For this review, take the finished solid that the model builds, in its own axes (mm). A direction names the side the tool comes from. Coordinates: 2 decimals unless noted, no trailing zeros. Order: outer loops, then holes, each group sorted by start corner. A loop starts at its lowest first (then second) coordinate and runs counter-clockwise, first axis right, second up. Notation, with made-up numbers: (84.5, 30) -> (108.5, 30) arc R38 ccw to (108.5, 68) -> close; hole circle Ø3 at (65, 12). An arc over 180 degrees is marked (long way). Return JSON: item names as keys, results as strings. Group by question number.
Item 1: Take a section at B-B (z = -6). Write out the cut boundary in (x, y), then the cut area to 3 significant figures.
Item 2: Take a section at D-D (x = -1). Write out the cut boundary in (y, z), then the cut area to 3 significant figures.
Item 3: Machinability: for faces 5 (the flat face through (0, 10, -5)), 6 (the cylindrical face through (-20.839, -4.213, -5.549)), 7 (the cylindrical face through (-41, 0, 2)), which of the approach directions +Z, -Z, +X, -X, +Y, -Y give a long, thin tool a straight path to every point of the face, cutting with its end or side? Answer none if there is none.
Item 4: Take a section at A-A (x = -31). Write out the cut boundary in (y, z), then the cut area to 4 significant figures.
Item 5: Draft analysis for pull direction Y (two halves, no side actions). For faces 1 (the flat face through (-78, 18.5, -2)), 2 (the flat face through (-4, -13.5, -2)), 3 (the cylindrical face through (-166.33, 16.04, -0.35)), 4 (the flat face through (-29, -10, -2)), state which applies: +Y half, -Y half, draft (parallel to the pull), parting line (faces both ways), or undercut.
Item 6: Take a section at C-C (y = 0). Write out the cut boundary in (x, z).
Item 7: For line 1 along Y through (x, z) = (-12, 4.85); line 2 along X through (y, z) = (16.95, -1.5); line 3 along Y through (x, z) = (-48.5, -8.25), list the stretches that pass through material, from the lowest coordinate up.
Item 8: Insertion check: pin 1 (4.5 mm diameter, centred on x = -6, z = -6, fed in from -Y); pin 2 (2 mm diameter, centred on y = -6, z = 3, fed in from -X); pin 3 (6 mm diameter, centred on x = 4, y = 3.5, fed in from -Z). Each pin has a flat end and moves straight along its axis. Give the tip position at first contact, or say it passes through.
```python
from build123d import *

# Parameters (mm, degrees)
SKETCH_1_W          = 40
SKETCH_1_H          = 20
EXTRUDE_1_DEPTH     = 6
SKETCH_2_R          = 2.5
CUT_EXTRUDE_1_DEPTH = 24.151673806
EXTRUDE_START       = -15
EXTRUDE_2_OUTLINE_R = 11
EXTRUDE_2_DEPTH     = 15
EXTRUDE_START_2     = -8
SKETCH_5_R          = 11
SKETCH_5_R_2        = 10
EXTRUDE_3_DEPTH     = 8
SKETCH_8_W          = 15
SKETCH_8_H          = 5
EXTRUDE_4_DEPTH     = 200
SKETCH_9_W          = 4.403653586
SKETCH_9_H          = 3.736433346
EXTRUDE_5_DEPTH     = 15
SKETCH_13_W         = 64.67728996
SKETCH_13_H         = 18.524474632
CUT_EXTRUDE_2_DEPTH = 184.131783151
SKETCH_15_W         = 55.676477601
SKETCH_15_H         = 15
EXTRUDE_6_DEPTH     = 5
SKETCH_16_R         = 2.5
CUT_EXTRUDE_3_DEPTH = 10


# Read off the part's stored shape, not the designer's step: 凸台-拉伸2
with BuildPart() as part:
    # 草图1 → 凸台-拉伸1 (new body)
    with BuildSketch(Plane.XY):
        Rectangle(SKETCH_1_W, SKETCH_1_H)
    extrude(amount=EXTRUDE_1_DEPTH)

    # 草图2 → 切除-拉伸1 (cut, through all)
    with BuildSketch(Plane.XY.offset(6)):
        with Locations((10, 0)):
            Circle(SKETCH_2_R)
        with Locations((-1, 0)):
            Circle(SKETCH_2_R)
        with Locations((-12, 0)):
            Circle(SKETCH_2_R)
    extrude(amount=-CUT_EXTRUDE_1_DEPTH, mode=Mode.SUBTRACT)

    # 凸台-拉伸2 outline → 凸台-拉伸2 (add)
    with BuildSketch(Plane.XY.offset(6).offset(EXTRUDE_START)):
        with BuildLine():
            Line((20, 10), (20, 13.5))
            Line((20, 13.5), (-26.893967141, 13.5))
            Line((-26.893967141, 13.5), (-26.893967141, 13.384337644))
            ThreePointArc((-26.893967141, 13.384337644), (-45, 0), (-26.893967141, -13.384337644))
            Line((-26.893967141, -13.384337644), (-26.893967141, -13.5))
            Line((-26.893967141, -13.5), (20, -13.5))
            Line((20, -13.5), (20, -10))
            Line((20, -10), (-20, -10))
            Line((-20, -10), (-20, -8.660254038))
            ThreePointArc((-20, -8.660254038), (-17, 0), (-20, 8.660254038))
            Line((-20, 8.660254038), (-20, 10))
            Line((-20, 10), (20, 10))
        make_face()
        with Locations((-31, 0)):
            Circle(EXTRUDE_2_OUTLINE_R, mode=Mode.SUBTRACT)
    extrude(amount=EXTRUDE_2_DEPTH)

    # 草图5 → 凸台-拉伸3 (add)
    with BuildSketch(Plane.XY.offset(6).offset(EXTRUDE_START_2)):
        with Locations((-31, 0)):
            Circle(SKETCH_5_R)
        with Locations((-31, 0)):
            Circle(SKETCH_5_R_2, mode=Mode.SUBTRACT)
    extrude(amount=EXTRUDE_3_DEPTH)

    # 草图8 → 凸台-拉伸4 (add)
    with BuildSketch(Plane(origin=(20, 0, 0), x_dir=(0, 0, -1), z_dir=(1, 0, 0))):
        with Locations((1.5, 16)):
            Rectangle(SKETCH_8_W, SKETCH_8_H)
    extrude(amount=-EXTRUDE_4_DEPTH)

    # 草图9 → 凸台-拉伸5 (add, through all)
    with BuildSketch(Plane.XY.offset(6)):
        with Locations((-27.364497847, 13.796597935)):
            Rectangle(SKETCH_9_W, SKETCH_9_H)
    extrude(amount=-EXTRUDE_5_DEPTH)

    # 草图13 → 切除-拉伸2 (cut, through all)
    with BuildSketch(Plane(origin=(0, 18.5, 0), x_dir=(1, 0, 0), z_dir=(0, 1, 0))):
        with Locations((-150.772464122, 3.262237316)):
            Rectangle(SKETCH_13_W, SKETCH_13_H)
    extrude(amount=-CUT_EXTRUDE_2_DEPTH, mode=Mode.SUBTRACT)

    # 草图15 → 凸台-拉伸6 (add)
    with BuildSketch(Plane(origin=(0, 18.5, 0), x_dir=(1, 0, 0), z_dir=(0, 1, 0))):
        with Locations((-146.272057942, 1.5)):
            Rectangle(SKETCH_15_W, SKETCH_15_H)
    extrude(amount=-EXTRUDE_6_DEPTH)

    # 草图16 → 切除-拉伸3 (cut)
    with BuildSketch(Plane(origin=(0, 18.5, 0), x_dir=(1, 0, 0), z_dir=(0, 1, 0))):
        with Locations(Location((-164.110296743, 1.5, 0), (0, 0, 270))):
            Circle(SKETCH_16_R)
    extrude(amount=-CUT_EXTRUDE_3_DEPTH, mode=Mode.SUBTRACT)


solid = part.part
```
Findings below:
{
 "1": {"outline": "(-174.11, 13.5) -> (-34.71, 13.5) arc R14 ccw (long way) to (-26.89, -13.38) -> (-26.89, -13.5) -> (20, -13.5) -> (20, -10) -> (-20, -10) -> (-20, -8.66) arc R14 ccw to (-20, 8.66) -> (-20, 10) -> (20, 10) -> (20, 18.5) -> (-174.11, 18.5) -> close; hole circle Ø22 at (-31, 0)", "area": "1,510 mm2"},
 "2": {"outline": "(-13.5, -9) -> (-10, -9) -> (-10, 0) -> (-2.5, 0) -> (-2.5, 6) -> (-13.5, 6) -> close; (2.5, 0) -> (10, 0) -> (10, -9) -> (18.5, -9) -> (18.5, 6) -> (2.5, 6) -> close", "area": "270 mm2"},
 "3": {"face 5": "-Z, +X", "face 6": "-Z", "face 7": "+Z, -Z"},
 "4": {"outline": "(-14, -9) -> (-11, -9) -> (-11, -2) -> (-10, -2) -> (-10, 6) -> (-14, 6) -> close; (10, -2) -> (11, -2) -> (11, -9) -> (18.5, -9) -> (18.5, 6) -> (10, 6) -> close", "area": "173.5 mm2"},
 "5": {"face 1": "+Y half", "face 2": "-Y half", "face 3": "draft", "face 4": "undercut"},
 "6": {"outline": "(-45, -9) -> (-42, -9) -> (-42, -2) -> (-41, -2) -> (-41, 6) -> (-45, 6) -> close; (-21, -2) -> (-20, -2) -> (-20, -9) -> (-17, -9) -> (-17, 0) -> (-14.5, 0) -> (-14.5, 6) -> (-21, 6) -> close; (-9.5, 0) -> (-3.5, 0) -> (-3.5, 6) -> (-9.5, 6) -> close; (1.5, 0) -> (7.5, 0) -> (7.5, 6) -> (1.5, 6) -> close; (12.5, 0) -> (20, 0) -> (20, 6) -> (12.5, 6) -> close"},
 "7": {"line 1": "y = -13.5 to -2.5, 2.5 to 18.5", "line 2": "x = -174.11 to -166.61, -161.61 to 20", "line 3": "y = 13.5 to 18.5"},
 "8": {"pin 1": "stops at y = -13.5", "pin 2": "stops at x = -44.08", "pin 3": "stops at z = 0"}
}
